Autodesk Inventor part; units mm, degrees
ref_plane "YZ Plane" through (0, 0, 0) normal (1, 0, 0) x (0, 1, 0)
ref_plane "XZ Plane" through (0, 0, 0) normal (0, 1, 0) x (-1, 0, 0)
ref_plane "XY Plane" through (0, 0, 0) normal (0, 0, 1) x (1, 0, 0)
sketch "Sketch1" plane through (0, 0, 0) normal (1, 0, 0) x (0, 1, 0)
  circle A0 centre (-9.7574, -19.7073) radius 1.55 construction
  circle A1 centre (0, 0) radius 1.55 construction
  circle A2 centre (-9.7574, -19.7073) radius 2.65
  circle A3 centre (0, 0) radius 2.65
  line L0 (-6.0684, -24.2876) -> (12.7398, 12.1607) construction
  arc A4 (-12.2239, -24.4871) -> (-4.9776, -22.1738) centre (-9.7574, -19.7073) ccw
  circle A5 centre (0, 0) radius 5.7448
  line L1 (-4.9776, -22.1738) -> (5.1052, -2.6344)
  arc A6 (-4.9776, -22.1738) -> (-12.2239, -24.4871) centre (-9.7574, -19.7073) ccw
  line L2 (-14.5372, -17.2408) -> (-5.1904, 2.4623)
  line L3 (0, 0) -> (0, -27.0135) construction
  line L4 (0, 0) -> (-9.7574, -19.7073) construction
  point P0 (-10.1101, -25.5779)
  dimension "d0" = 5.3
  dimension "d1" = 5.3
  dimension "d3" = 11.4897
  dimension "d4" = 5.3787
  dimension "d5" = 21.8076
  dimension "d6" = 21.9875
extrude "Extrusion1" add sketch "Sketch1" along normal blind 19
sketch "Sketch2" plane through (19, 0, 0) normal (1, 0, 0) x (0, 0, -1)
  arc A0 (17.2408, -14.5372) -> (22.1738, -4.9776) centre (19.7073, -9.7574) ccw
  line L0 (22.1738, -4.9776) -> (2.6344, 5.1052)
  arc A1 (2.6344, 5.1052) -> (-2.4623, -5.1904) centre (0, 0) ccw
  line L1 (-2.4623, -5.1904) -> (17.2408, -14.5372) construction
  circle A2 centre (19.7073, -9.7574) radius 2.65 construction
  circle A3 centre (0, 0) radius 2.65 construction
  circle A4 centre (19.7073, -9.7574) radius 2.65 construction
  line L2 (-0.0042, 0.0021) -> (19.7073, -9.7574) construction
  circle A5 centre (12.4634, 13.9146) radius 1
  circle A6 centre (12.4634, 13.9146) radius 4
  line L3 (9.7462, 16.85) -> (-3.9025, 4.2159)
  arc A7 (2.6344, 5.1052) -> (-2.4623, -5.1904) centre (0, 0) ccw
  line L4 (16.2172, 15.2963) -> (24.7549, -7.8995)
  line L5 (-12.5084, -12.3162) -> (6.9664, 27.0174)
  point P0 (-3.9025, 4.2159)
  dimension "d11" = 2
  dimension "d12" = 8
  dimension "d20" = 18
  dimension "d21" = 10.7401
extrude "Extrusion2" [suppressed]
sketch "Sketch3" plane through (19, 0, 0) normal (1, 0, 0) x (0, 0, -1)
  circle A0 centre (12.4634, 13.9146) radius 1
  circle A1 centre (12.4634, 13.9146) radius 2.5
  point P0 (0, 0)
  dimension "d15" = 5
extrude "Extrusion3" [suppressed]
sketch "Sketch4" plane through (19, 0, 0) normal (1, 0, 0) x (0, 0, -1)
  arc A0 (2.6344, 5.1052) -> (-2.4623, -5.1904) centre (0, 0) ccw
  line L0 (-2.4623, -5.1904) -> (17.2408, -14.5372)
  arc A1 (17.2408, -14.5372) -> (22.1738, -4.9776) centre (19.7073, -9.7574) ccw
  line L1 (22.1738, -4.9776) -> (2.6344, 5.1052)
  circle A2 centre (19.7073, -9.7574) radius 2.65
  circle A3 centre (0, 0) radius 2.65
  arc A4 (2.6344, 5.1052) -> (-2.4623, -5.1904) centre (0, 0) ccw
  arc A5 (17.2408, -14.5372) -> (22.1738, -4.9776) centre (19.7073, -9.7574) ccw
  arc A6 (2.6344, 5.1052) -> (22.1738, -4.9776) centre (18.6478, 12.1635) ccw
  dimension "d22" = 17.5
extrude "Extrusion4" cut sketch "Sketch4" against normal through all contours L1 A6
fillet "Fillet1" radius 3 2 edges at (9.5, -4.9776, -22.1738) (9.5, 5.1052, -2.6344)
properties part number "Kauri modular camera mount spacer micro outside" material "Brass, Soft Yellow"
Input: part model. Units: mm. Frame: model coordinates. Give positions to 0.01 mm unless a question says otherwise; leave off trailing zeros. Order: outer loops, then holes, each group sorted by start corner. A loop starts at its lowest first (then second) coordinate and runs counter-clockwise, first axis right, second up. Notation, with made-up numbers: (30, 74.25) - (80, 74.25) arc R23 ccw to (80, 91.25) - close; hole circle Ø8 at (12, 53). An arc over 180 degrees is marked (long way). One line per item, written item: value.
1. Cut plane A-A, the plane z = 0. Output: boundary loops of the cut face in (x, y).
Determined:
outline: (0, -6.36) - (19, -6.36) - (19, -2.65) - (0, -2.65) - close; (0, 2.65) - (19, 2.65) - (19, 5.74) - (0, 5.74) - close
2. Cut plane C-C, the plane x = 8. Give the number of separate pieces and of enclosed holes in the cut face, and give its area (3 significant figures).
Determined:
separate pieces: 1
enclosed holes: 2
area: 239 mm2
3. Draft query along Z for faces 1 (the face through (9.37, -9.93, -7.53)), 2 (the face through (0, -5, -10)), 3 (the face through (9.37, -11.71, -21.5)). Return one class per face: released by +Z, released by -Z, zero draft, split by the parting line, or undercut.
Determined:
face 1: released by +Z
face 2: zero draft
face 3: undercut
4. Pin query (flat end, axial travel): pin 1 Ø10 at (x, y) = (7.5, -11) entering from +Z; pin 2 Ø5 at (y, z) = (-9.76, -19.71) entering from +X; pin 3 Ø2 at (x, z) = (16.5, -2.5) entering from +Y. Return the tip coordinate at first contact, or that it passes through.
Determined:
pin 1: z = 0.76
pin 2: through
pin 3: y = 5.52
5. Cut plane D-D, the plane y = 3.5. Output: boundary loops of the cut face in (x, z), and give its area (3 significant figures).
Determined:
outline: (0, -3.44) - (19, -3.44) - (19, 4.56) - (0, 4.56) - close
area: 152 mm2
6. Cut plane B-B, the plane y = -8.25. Output: boundary loops of the cut face in (x, z), and give its area (3 significant figures).
Determined:
outline: (0, -24.87) - (19, -24.87) - (19, -21.89) - (0, -21.89) - close; (0, -17.53) - (19, -17.53) - (19, -3.99) - (0, -3.99) - close
area: 314 mm2
7. Line query: probe 1 along Z at (x, y) = (11, 0); probe 2 along Y at (x, z) = (13.5, -18); probe 3 along Y at (x, z) = (8.75, 1.5). Output: solid intervals per line, ascending.
Determined:
probe 1: -6.07 to -2.65, 2.65 to 5.74
probe 2: -14.86 to -11.78, -7.73 to -5.32
probe 3: -5.65 to -2.18, 2.18 to 5.55
